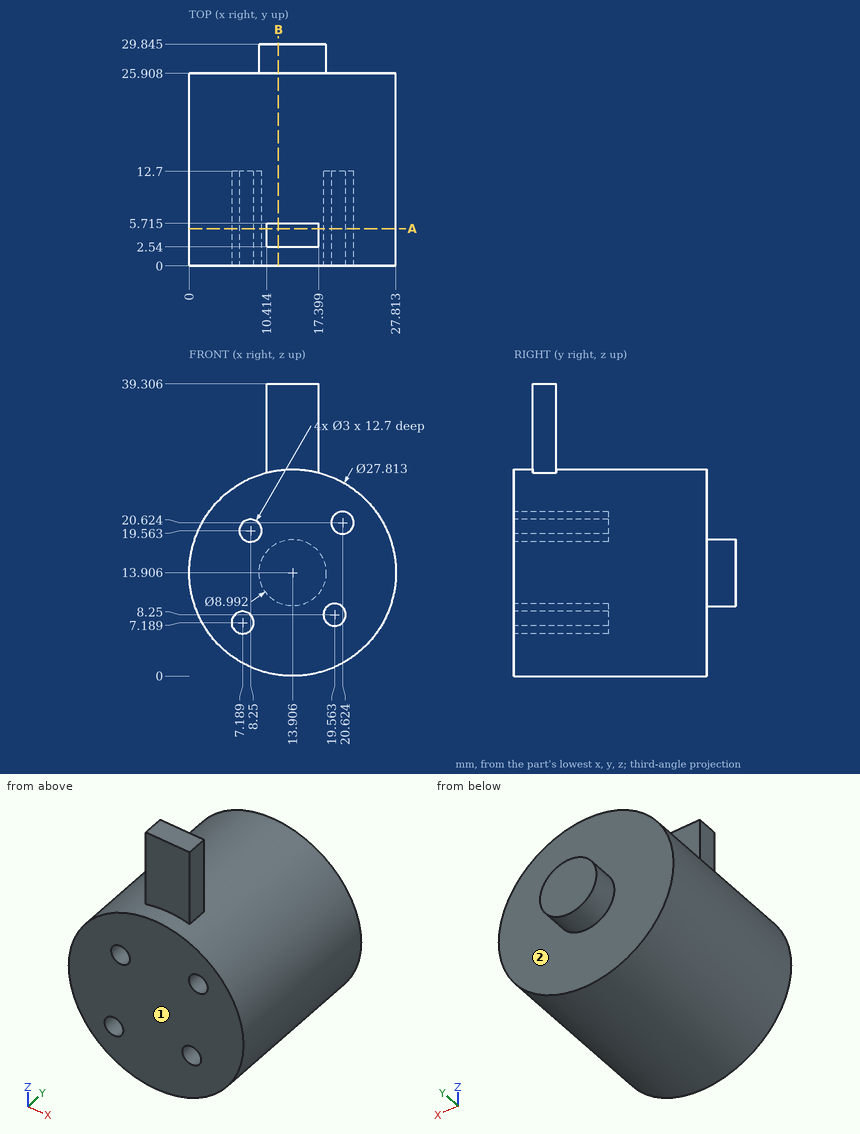
Drawing for the job (mm, zero at the part's lowest x, y, z). A direction names the side the tool comes from. Give positions to 0.01 mm unless a question says otherwise; leave off trailing zeros. Order: outer loops, then holes, each group sorted by start corner. A loop starts at its lowest first (then second) coordinate and runs counter-clockwise, first axis right, second up. Notation, with made-up numbers: M 48.25,31.5 L 67.25,31.5 A17 cw 67.25,35.5 Z; hole C -2,-15 d10. An arc over 180 degrees is marked long. Write item = value, one per line. Start each with the question number.
(1) Slice it at A-A on y = 5. State how many separate pieces and enclosed holes the cut face has.
(2) Which spindle directions (+Z, -Z, +X, -X, +Y, -Y) get a long thin tool onto all of the face, cutting with end or side? Do the marked faces 1 and 2. Say none if no direction does.
(3) Pin check, flat tips, straight feed: pin 1 Ø2.5 at (x, z) = (20, 8) entering from -Y; pin 2 Ø1 at (y, z) = (11.5, 7.5) entering from -X; pin 3 Ø1 at (x, y) = (5.5, 12) entering from +Z; pin 4 Ø1.6 at (y, z) = (4, 34) entering from +X. Stop position of each tip, or through.
(4) Slice it at B-B on x = 12. Write the cut outline in (y, z) (1 decimal).
(5) Probe L1, parallel to Z at x = 8.5, y = 6.75 (1 decimal); L2, parallel to Y at x = 6, z = 10; L3, parallel to Y at x = 18.75, z = 8. List the from-to ranges inside material, lowest first. Write a range as [from, to].
Responses:
q1.separate_pieces = 1
q1.enclosed_holes = 4
q2.face_1 = +Z, -Z, +X, -X, -Y
q2.face_2 = +Y
q3.pin_1 = 0
q3.pin_2 = 1.32
q3.pin_3 = 25.35
q3.pin_4 = 17.4
q4.outline = M 0,0.1 L 25.9,0.1 L 25.9,9.8 L 29.8,9.8 L 29.8,18 L 25.9,18 L 25.9,27.7 L 5.7,27.7 L 5.7,39.3 L 2.5,39.3 L 2.5,27.7 L 0,27.7 Z
q5.L1 = [1.1, 6.5], [7.9, 18.1], [21, 26.7]
q5.L2 = [0, 25.91]
q5.L3 = [12.7, 25.91]
